Build history of the part. All positions in model axes, mm. Face numbers are marked on the shaded views. A direction names the side the tool comes from. Round coordinates to 2 decimals unless told otherwise and drop trailing zeros. Write each loop counter-clockwise with the first axis right and the second up, starting at its lowest first coordinate (ties: lowest second). Pieces come first, ordered by that corner, then holes. Notation, with made-up numbers: (-25, 0.25) -> (4, 0.25) arc R26 ccw to (4, 34.25) -> close; hole circle Ø11 at (5, -27.5). An arc over 180 degrees is marked (long way). Answer as CSV lines item,"result".
from build123d import *

# Parameters (mm, degrees)
SKETCH2_R          = 0.4
CUT_EXTRUDE1_DEPTH = 4


with BuildPart() as part:
    # Sketch1 → Revolve1 (revolve)
    with BuildSketch(Plane.XY):
        with BuildLine():
            Line((0, 1.8), (-0.8, 1))
            Line((-0.8, 1), (-7.711324865, 1))
            Line((-7.711324865, 1), (-8, 0.5))
            Line((-8, 0.5), (-21.5, 0.5))
            Line((-21.5, 0.5), (-22, 1))
            Line((-22, 1), (-22, 1.423349476))
            ThreePointArc((-22, 1.423349476), (-21.89667667, 1.72773019), (-21.629409523, 1.906312389))
            Line((-21.629409523, 1.906312389), (-20.346749895, 2.25))
            ThreePointArc((-20.346749895, 2.25), (-19.766015063, 2.23084248), (-19.293965425, 1.892037087))
            ThreePointArc((-19.293965425, 1.892037087), (-18.942739815, 1.603349869), (-18.5, 1.5))
            Line((-18.5, 1.5), (-15, 1.5))
            ThreePointArc((-15, 1.5), (-14.434314575, 1.734314575), (-14.2, 2.3))
            Line((-14.2, 2.3), (-14.2, 2.8))
            Line((-14.2, 2.8), (-14, 3))
            Line((-14, 3), (-13, 3))
            Line((-13, 3), (-13, 2))
            Line((-13, 2), (0, 2))
            Line((0, 2), (0, 1.8))
        make_face()
    revolve(axis=Axis((0, 0, 0), (-1, 0, 0)))

    # Sketch2 → Cut-Extrude1 (cut, through all)
    with BuildSketch(Plane(origin=(0, 0, 0), x_dir=(1, 0, 0), z_dir=(0, 1, 0))):
        with Locations(Location((-7, 0, 0), (0, 0, 180))):  # turned: the seam where the file's is
            Circle(SKETCH2_R)
    extrude(amount=CUT_EXTRUDE1_DEPTH, mode=Mode.SUBTRACT)


solid = part.part
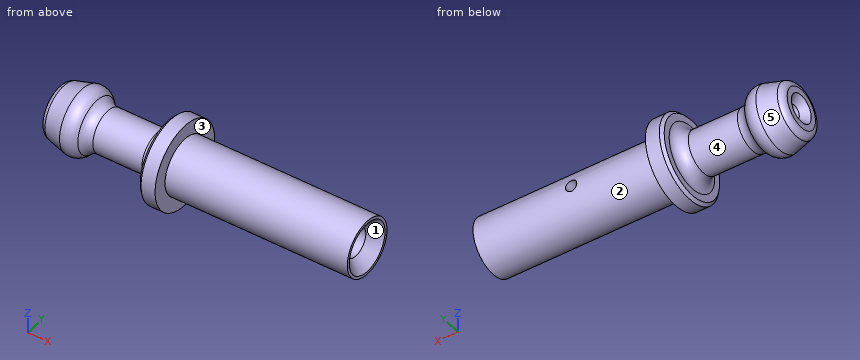
1. Which spindle directions (+Z, -Z, +X, -X, +Y, -Y) get a long thin tool onto all of the face, cutting with end or side? Do the marked faces 4 and 5. Say none if no direction does.
Results found:
face 4,"none"
face 5,"-X"
2. Cut at B-B, the plane z = 0. Count the separate pieces of the cut face and the enclosed holes in it, then the cut area to 3 significant figures.
Results found:
separate pieces,"3"
enclosed holes,"0"
area,"54.6 mm2"
3. Cut at C-C, the plane x = -17.75. Write the cut outline in (y, z).
Results found:
outline,"circle Ø3 at (0, 0); hole circle Ø1 at (0, 0)"
4. Probe line 1 along Z through (x, y) = (-13.25, 0); line 2 along Y through (x, z) = (-15.25, 0). List the from-to ranges inside material, lowest first.
Results found:
line 1,"z = -3 to -0.5, 0.5 to 3"
line 2,"y = -1.5 to -0.5, 0.5 to 1.5"
5. Mould opens along Z. For the marked faces 1, 2 and 3 say: +Z half, -Z half, draft (parallel to the pull), parting line (faces both ways), or undercut.
Results found:
face 1,"undercut"
face 2,"parting line"
face 3,"draft"
6. Drop flat-ended pins along their axis: pin 1 Ø1.5 at (x, z) = (-15.5, 1.5) entering from +Y; pin 2 Ø1.5 at (y, z) = (0.5, 0.5) entering from -X; pin 3 Ø1 at (x, y) = (-4.5, 0.5) entering from +Z; pin 4 Ø2.5 at (y, z) = (0, 0) entering from +X. Give the stop position or say it passes through.
Results found:
pin 1,"stops at y = 1.3"
pin 2,"stops at x = -22"
pin 3,"stops at z = 2"
pin 4,"stops at x = -0.55"
7. Cut at D-D, the plane x = -7. Write the cut outline in (y, z), then the cut area to 3 significant figures.
Results found:
outline,"(0.92, -0.4) arc R1 cw (long way) to (0.92, 0.4) -> (1.96, 0.4) arc R2 ccw (long way) to (1.96, -0.4) -> close"
area,"8.61 mm2"
8. Cut at A-A, the plane x = -1.25. Write the cut outline in (y, z).
Results found:
outline,"circle Ø4 at (0, 0); hole circle Ø2 at (0, 0)"
